Verification items for the finished model (mm, model axes). A direction names the side the tool comes from. Give positions to 0.01 mm unless a question says otherwise; leave off trailing zeros. Loops run counter-clockwise (first coordinate to the right, second up) from the corner with the lowest first, then second, coordinate; pieces in that order, holes last. Notation, with made-up numbers: (-23, -7.5) - (14, -7.5) arc R30 cw to (14, 16.5) - close; hole circle Ø1 at (73, 70). An arc over 180 degrees is marked (long way). Put each result on its own line as item: value. Start each with the question number.
```python
from build123d import *

# Parameters (mm, degrees)
SZKIC1_W                       = 44
SZKIC1_H                       = 20
DODANIE_WYCI_GNI_CIE1_DEPTH    = 40
SZKIC3_R                       = 11
WYTNIJ_WYCI_GNI_CIE2_DEPTH     = 50.839743178
SZKIC4_R                       = 14
WYTNIJ_WYCI_GNI_CIE3_DEPTH     = 11
OTW_R_GWINTOWANY_M5X0_81_D     = 4.2
OTW_R_GWINTOWANY_M5X0_81_DEPTH = 25
OTW_R_GWINTOWANY_M5X0_81_TIP   = 1.2618073
SZKIC5_W                       = 1.3
SZKIC5_H                       = 0.7


with BuildPart() as part:
    # Szkic1 → Dodanie-wyciągnięcie1 (new body)
    with BuildSketch(Plane(origin=(0, 0, 0), x_dir=(1, 0, 0), z_dir=(0, 1, 0))):
        Rectangle(SZKIC1_W, SZKIC1_H)
    extrude(amount=DODANIE_WYCI_GNI_CIE1_DEPTH)

    # Szkic3 → Wytnij-wyciągnięcie2 (cut, through all)
    with BuildSketch(Plane.XY.offset(10)):
        with Locations((0, 16.5)):
            Circle(SZKIC3_R)
    extrude(amount=-WYTNIJ_WYCI_GNI_CIE2_DEPTH, mode=Mode.SUBTRACT)

    # Szkic4 → Wytnij-wyciągnięcie3 (cut)
    with BuildSketch(Plane.XY.offset(10)):
        with Locations((0, 16.5)):
            Circle(SZKIC4_R)
    extrude(amount=-WYTNIJ_WYCI_GNI_CIE3_DEPTH, mode=Mode.SUBTRACT)

    # Otwór gwintowany M5x0.81
    with Locations(Plane(origin=(0, 40, 0), x_dir=(1, 0, 0), z_dir=(0, 1, 0))):
        with Locations((17, 5), (17, -5), (-17, -5), (-17, 5)):
            Hole(OTW_R_GWINTOWANY_M5X0_81_D / 2, depth=OTW_R_GWINTOWANY_M5X0_81_DEPTH)
            with Locations((0, 0, -(OTW_R_GWINTOWANY_M5X0_81_DEPTH + OTW_R_GWINTOWANY_M5X0_81_TIP / 2))):  # 118° drill point
                Cone(0, OTW_R_GWINTOWANY_M5X0_81_D / 2, OTW_R_GWINTOWANY_M5X0_81_TIP, mode=Mode.SUBTRACT)

    # Szkic5 → Wycięcie-obrót1 (revolve, cut)
    with BuildSketch(Plane(origin=(0, 0, 0), x_dir=(0, 0, -1), z_dir=(1, 0, 0)), mode=Mode.PRIVATE) as wyci_cie_obr_t1_sk:
        with Locations((-7.65, 2.15)):
            Rectangle(SZKIC5_W, SZKIC5_H)
    revolve(wyci_cie_obr_t1_sk.sketch.rotate(Axis((0, 16.5, 9.294649117), (0, 0, 1)), 90), axis=Axis((0, 16.5, 9.294649117), (0, 0, 1)), mode=Mode.SUBTRACT)


solid = part.part
```
1) Section check A-A, the plane x = 0. Enter the section's corners in (y, z), plus the area to 3 significant figures.
2) Draft check along Z on faces 1 (the face through (0, 33, 10)), 2 (the face through (22, 20, 0)), 3 (the face through (-3.19, 2.15, 7.64)). Enter one of: pulls with the +Z half, pulls with the -Z half, needs draft (parallel to the pull), parting line crosses it, or undercut.
3) Section check D-D, the plane y = 10. Enter the section's corners in (x, z), plus the area to 3 significant figures.
4) Set-up check for faces 4 (the face through (15.06, 27.33, 5.8)), 5 (the face through (-3.03, 2.83, 3.06)), 6 (the face through (12, 9, 7)): record each of +Z, -Z, +X, -X, +Y, -Y from which the full face is reachable in a straight line by a thin tool's end or side.
5) Section check C-C, the plane z = 0.5. Enter the section's corners in (x, y), plus the area to 3 significant figures.
6) Depth check by flat-ended pin: P1, Ø14, axis at x = 0.5, y = 21.5, coming from the +Z side. Enter the tip coordinate at first touch or a pass-through.
7) Section check B-B, the plane y = 21. Enter the section's corners in (x, z), plus the area to 3 significant figures.
8) Scan lines: line 1 along Y through (x, z) = (0, 9.4); line 2 along Y through (x, z) = (0, -4.75); line 3 along X through (y, z) = (14.5, 5.25). Record each from-to range of solid material in increasing order. Write a range as from..to.
Results are:
1. outline: (0, -10) - (5.5, -10) - (5.5, -1) - (2.5, -1) - (2.5, 7) - (1.8, 7) - (1.8, 8.3) - (2.5, 8.3) - (2.5, 10) - (0, 10) - close; (27.5, -10) - (40, -10) - (40, 10) - (30.5, 10) - (30.5, 8.3) - (31.2, 8.3) - (31.2, 7) - (30.5, 7) - (30.5, -1) - (27.5, -1) - close
1. area: 292 mm2
2. face 1: pulls with the +Z half
2. face 2: needs draft
2. face 3: undercut
3. outline: (-22, -10) - (-8.87, -10) - (-8.87, -1) - (-12.4, -1) - (-12.4, 7) - (-13.18, 7) - (-13.18, 8.3) - (-12.4, 8.3) - (-12.4, 10) - (-22, 10) - close; (8.87, -10) - (22, -10) - (22, 10) - (12.4, 10) - (12.4, 8.3) - (13.18, 8.3) - (13.18, 7) - (12.4, 7) - (12.4, -1) - (8.87, -1) - close
3. area: 445 mm2
4. face 4: +Y
4. face 5: +Z
4. face 6: none
5. outline: (-22, 0) - (22, 0) - (22, 40) - (-22, 40) - close; hole circle Ø28 at (0, 16.5)
5. area: 1,140 mm2
6. P1: stops at z = -1
7. outline: (-22, -10) - (-10.04, -10) - (-10.04, -1) - (-13.26, -1) - (-13.26, 7) - (-13.99, 7) - (-13.99, 8.3) - (-13.26, 8.3) - (-13.26, 10) - (-22, 10) - close; (10.04, -10) - (22, -10) - (22, 10) - (13.26, 10) - (13.26, 8.3) - (13.99, 8.3) - (13.99, 7) - (13.26, 7) - (13.26, -1) - (10.04, -1) - close; hole circle Ø4.2 at (-17, -5); hole circle Ø4.2 at (-17, 5); hole circle Ø4.2 at (17, -5); hole circle Ø4.2 at (17, 5)
7. area: 350 mm2
8. line 1: y = 0..2.5, 30.5..40
8. line 2: y = 0..5.5, 27.5..40
8. line 3: x = -22..-18.24, -15.76..-13.86, 13.86..15.76, 18.24..22
